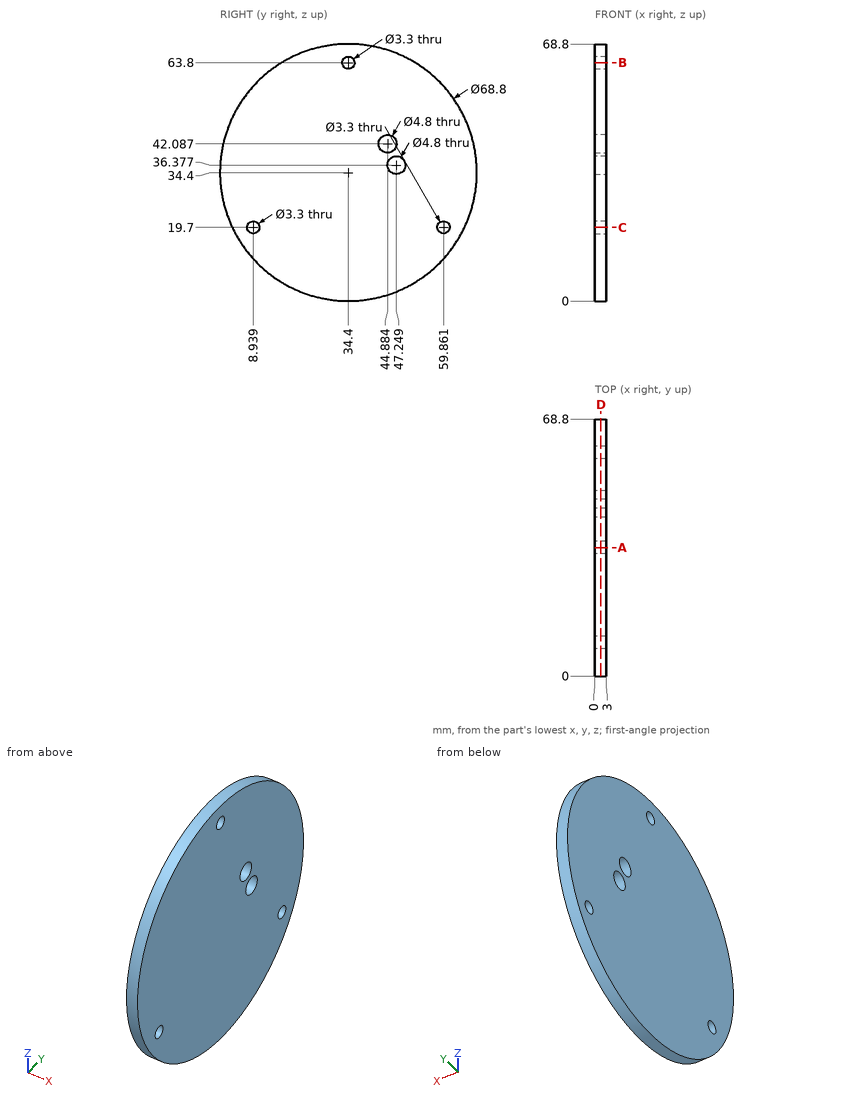
Can you work these out from the drawing? Everything is in mm from the part's minimum corner. Coordinates: 2 decimals unless noted, no trailing zeros. Loops run counter-clockwise (first coordinate to the right, second up) from the corner with the lowest first, then second, coordinate; pieces in that order, holes last. Notation, with made-up numbers: (-17, 2.5) - (31, 2.5) arc R30 cw to (31, 41.5) - close; hole circle Ø7 at (29, -8). An arc over 180 degrees is marked (long way). Answer as CSV lines item,"result".
Q1. If we section it at A-A, the plane y = 34.4: Write out the boundary of the cut face in (x, z).
Response:
outline,"(0, 0) - (3, 0) - (3, 62.15) - (0, 62.15) - close; (0, 65.45) - (3, 65.45) - (3, 68.8) - (0, 68.8) - close"
Q2. If I drill on L1, parallel to Y at x = 2.2, z = 19.7; L2, parallel to Z at x = 2.65, y = 47.5 (1 decimal); L3, parallel to Y at x = 1.65, z = 63.8, over which ranges is the centre line in solid material (lowest first)? Write a range as [from, to].
Response:
L1,"[3.3, 7.29], [10.59, 58.21], [61.51, 65.5]"
L2,"[2.6, 34], [38.8, 66.2]"
L3,"[16.54, 32.75], [36.05, 52.26]"
Q3. If we section it at D-D, the plane x = 1.6: Write out the boundary of the cut face in (y, z).
Response:
outline,"circle Ø68.8 at (34.4, 34.4); hole circle Ø3.3 at (8.94, 19.7); hole circle Ø3.3 at (34.4, 63.8); hole circle Ø4.8 at (44.88, 42.09); hole circle Ø4.8 at (47.25, 36.38); hole circle Ø3.3 at (59.86, 19.7)"
Q4. If we section it at C-C, the plane z = 19.7: Write out the boundary of the cut face in (x, y), and give its area (3 significant figures).
Response:
outline,"(0, 3.3) - (3, 3.3) - (3, 7.29) - (0, 7.29) - close; (0, 10.59) - (3, 10.59) - (3, 58.21) - (0, 58.21) - close; (0, 61.51) - (3, 61.51) - (3, 65.5) - (0, 65.5) - close"
area,"167 mm2"
Q5. For pin 1 (1.5 mm diameter, centred on x = 2, z = 57, fed in from -Y); pin 2 (2 mm diameter, centred on y = 17.5, z = 28, fed in from -X); pin 3 (1 mm diameter, centred on x = 1, z = 9.5, fed in from +Y), each with a flat end and sliding along its axis, tell me the tip position at first contact or that it passes through.
Response:
pin 1,"y = 7.83"
pin 2,"x = 0"
pin 3,"y = 58.65"
Q6. If we section it at B-B, the plane z = 63.8: Write out the boundary of the cut face in (x, y).
Response:
outline,"(0, 16.54) - (3, 16.54) - (3, 32.75) - (0, 32.75) - close; (0, 36.05) - (3, 36.05) - (3, 52.26) - (0, 52.26) - close"
